Verification items for the finished model (mm, model axes). Face numbers are marked on the shaded views. A direction names the side the tool comes from. Round coordinates to 2 decimals unless told otherwise and drop trailing zeros. Order: outer loops, then holes, each group sorted by start corner. A loop starts at its lowest first (then second) coordinate and runs counter-clockwise, first axis right, second up. Notation, with made-up numbers: M 33.25,64 L 52.25,64 A22 ccw 52.25,90 Z; hole C -15.75,16 d7. An arc over 180 degrees is marked long. Answer as a JSON object with one key per item and string values. Group by question number.
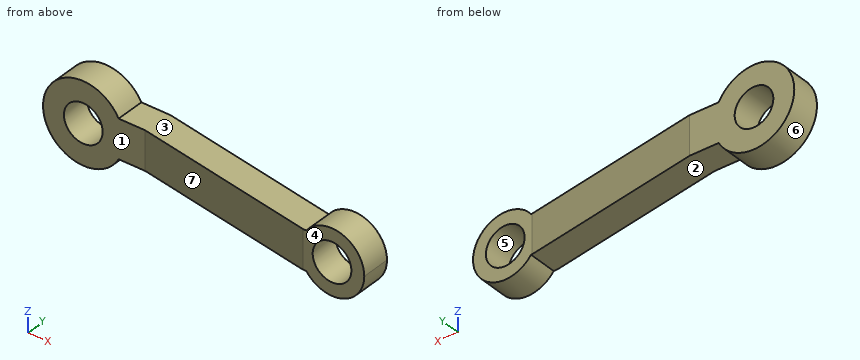
```python
from build123d import *

# Parameters (mm, degrees)
F0_R     = 6
F1_DEPTH = 25
F3_DEPTH = 12.5


with BuildPart() as f1:
    # F0 (on Front) → F1 (new body)
    with BuildSketch(Plane.XZ):
        with BuildLine():
            ThreePointArc((10.965856, -6), (12.110392, -3.096514), (12.5, 0))
            ThreePointArc((12.5, 0), (12.110392, 3.096514), (10.965856, 6))
            ThreePointArc((10.965856, 6), (-12.5, 0), (10.965856, -6))
        make_face()
        Circle(F0_R, mode=Mode.SUBTRACT)
        with BuildLine():
            ThreePointArc((10.965856, 6), (12.110392, 3.096514), (12.5, 0))
            ThreePointArc((12.5, 0), (12.110392, -3.096514), (10.965856, -6))
            Line((10.965856, -6), (77, -6))
            ThreePointArc((77, -6), (75, 0), (77, 6))
            Line((77, 6), (10.965856, 6))
        make_face()
        with BuildLine():
            ThreePointArc((95, 0), (88.162278, 9.486833), (77, 6))
            ThreePointArc((77, 6), (75, 0), (77, -6))
            ThreePointArc((77, -6), (88.162278, -9.486833), (95, 0))
        make_face()
        with Locations((85, 0)):
            Circle(F0_R, mode=Mode.SUBTRACT)
    extrude(amount=F1_DEPTH)

    # F2 (on Top) → F3 (intersect, symmetric)
    with BuildSketch(Plane.XY):
        Polygon((20, 0), (-12.5, 0), (-12.5, -9), (19.212602, -9), (75.92079, -18.999184), (95, -18.999184), (95, -9.999184), (76.708188, -9.999184), align=None)
    extrude(amount=F3_DEPTH, both=True, mode=Mode.INTERSECT)


solid = f1.part
```
Q1. Cross-section at C-C, the plane x = 0. Record the cut outline in (y, z), then the cut area to 3 significant figures.
Q2. Gauge pin test, flat ends, axial feed: pin 1 Ø1 at (x, z) = (10.5, 2) entering from -Y; pin 2 Ø6 at (y, z) = (-9.5, 4.5) entering from +X; pin 3 Ø10 at (x, z) = (47.5, 6) entering from +Y; pin 4 Ø11 at (x, z) = (0, 0) entering from -Y. Record the tip position at first contact, or that the pin passes through.
Q3. Cross-section at B-B, the plane z = 2.75. Record the cut outline in (x, y).
Q4. Cross-section at A-A, the plane x = 85. Record the cut outline in (y, z), then the cut area to 3 significant figures.
Q5. Release check for a two-part mould opening along X. For the marked faces 4, 5, 6 and 7 record: released by +X, released by -X, zero draft, split by the parting line, or undercut.
Q6. Thickness scan on line 1 (Z direction, x = 0, y = -5); line 2 (Y direction, x = 89, z = -5); line 3 (Z direction, x = 26, y = -7.5). Record the ranges inside material, lowest first. Write a range as from..to.
Q7. Tool access check on the marked faces 1, 2 and 3. Record the directions out of +Z, -Z, +X, -X, +Y, -Y that give a thin tool (end or side, any length) a straight path to the whole face; none if there is none.
Q8. Cross-section at D-D, the plane y = -13. Record the cut outline in (x, z).
Conclusion:
{
 "1": {"outline": "M -9,-12.5 L 0,-12.5 L 0,-6 L -9,-6 Z; M -9,6 L 0,6 L 0,12.5 L -9,12.5 Z", "area": "117 mm2"},
 "2": {"pin 1": "y = -9", "pin 2": "x = 94.88", "pin 3": "y = -3.97", "pin 4": "through"},
 "3": {"outline": "M -12.19,-9 L -5.33,-9 L -5.33,0 L -12.19,0 Z; M 5.33,-9 L 19.21,-9 L 75.92,-19 L 79.67,-19 L 79.67,-10 L 76.71,-10 L 20,0 L 5.33,0 Z; M 90.33,-19 L 94.61,-19 L 94.61,-10 L 90.33,-10 Z"},
 "4": {"outline": "M -19,-10 L -10,-10 L -10,-6 L -19,-6 Z; M -19,6 L -10,6 L -10,10 L -19,10 Z", "area": "72.0 mm2"},
 "5": {"face 4": "zero draft", "face 5": "undercut", "face 6": "split by the parting line", "face 7": "released by -X"},
 "6": {"line 1": "-12.5..-6, 6..12.5", "line 2": "-19..-10", "line 3": "-6..6"},
 "7": {"face 1": "+Z, -Z, -X, -Y", "face 2": "-Z, +Y, -Y", "face 3": "+Z, +Y, -Y"},
 "8": {"outline": "M 41.9,-6 L 77,-6 A10 ccw long 77,6 L 41.9,6 Z; hole C 85,0 d12"}
}
